```python
from build123d import *

# Parameters (mm, degrees)
SKETCH1_W                                         = 107.95
SKETCH1_H                                         = 101.6
SKETCH1_R                                         = 19.05
SKETCH1_R_2                                       = 2.15265
SKETCH1_W_2                                       = 6.604
SKETCH1_H_2                                       = 6.35
BOSS_EXTRUDE1_DEPTH                               = 6.604
F_10_32_TAPPED_HOLE1_D                            = 4.0386
F_10_32_TAPPED_HOLE1_DEPTH                        = 12.0396
F_10_32_TAPPED_HOLE1_TIP                          = 1.213317848
FILLET1_R                                         = 6.35
CSK_FOR_8_FLAT_HEAD_SOCKET_CAP_SCREW2_D           = 4.3053
CSK_FOR_8_FLAT_HEAD_SOCKET_CAP_SCREW2_CSINK_D     = 9.1186
CSK_FOR_8_FLAT_HEAD_SOCKET_CAP_SCREW2_CSINK_ANGLE = 82


with BuildPart() as part:
    # Sketch1 → Boss-Extrude1 (new body)
    with BuildSketch(Plane(origin=(0, 0, 0), x_dir=(0, 0, -1), z_dir=(1, 0, 0))):
        Rectangle(SKETCH1_W, SKETCH1_H)
        Circle(SKETCH1_R, mode=Mode.SUBTRACT)
        with Locations((-44.45, 31.75)):
            Circle(SKETCH1_R_2, mode=Mode.SUBTRACT)
        with Locations((-44.45, -31.75)):
            Circle(SKETCH1_R_2, mode=Mode.SUBTRACT)
        with Locations((44.45, 31.75)):
            Circle(SKETCH1_R_2, mode=Mode.SUBTRACT)
        with Locations((44.45, -31.75)):
            Circle(SKETCH1_R_2, mode=Mode.SUBTRACT)
        with Locations((-44.45, 41.275)):
            Rectangle(SKETCH1_W_2, SKETCH1_H_2, mode=Mode.SUBTRACT)
        with Locations((-44.45, 22.225)):
            Rectangle(SKETCH1_W_2, SKETCH1_H_2, mode=Mode.SUBTRACT)
        with Locations((-44.45, -22.225)):
            Rectangle(SKETCH1_W_2, SKETCH1_H_2, mode=Mode.SUBTRACT)
        with Locations((-44.45, -41.275)):
            Rectangle(SKETCH1_W_2, SKETCH1_H_2, mode=Mode.SUBTRACT)
        with Locations((44.45, 41.275)):
            Rectangle(SKETCH1_W_2, SKETCH1_H_2, mode=Mode.SUBTRACT)
        with Locations((44.45, 22.225)):
            Rectangle(SKETCH1_W_2, SKETCH1_H_2, mode=Mode.SUBTRACT)
        with Locations((44.45, -41.275)):
            Rectangle(SKETCH1_W_2, SKETCH1_H_2, mode=Mode.SUBTRACT)
        with Locations((44.45, -22.225)):
            Rectangle(SKETCH1_W_2, SKETCH1_H_2, mode=Mode.SUBTRACT)
    extrude(amount=BOSS_EXTRUDE1_DEPTH)

    # #10-32 Tapped Hole1
    with Locations(Plane(origin=(6.604, 0, 0), x_dir=(0, 0, -1), z_dir=(1, 0, 0))):
        with Locations((-23.622, 23.622), (23.622, 23.622), (-23.622, -23.622), (23.622, -23.622)):
            Hole(F_10_32_TAPPED_HOLE1_D / 2, depth=F_10_32_TAPPED_HOLE1_DEPTH)
            with Locations((0, 0, -(F_10_32_TAPPED_HOLE1_DEPTH + F_10_32_TAPPED_HOLE1_TIP / 2))):  # 118° drill point
                Cone(0, F_10_32_TAPPED_HOLE1_D / 2, F_10_32_TAPPED_HOLE1_TIP, mode=Mode.SUBTRACT)

    # Fillet1
    fillet1_edges = [part.edges().sort_by_distance(p)[0] for p in [
        (3.302, -50.8, -53.975),
        (3.302, -50.8, 53.975),
        (3.302, 50.8, 53.975),
        (3.302, 50.8, -53.975),
    ]]
    fillet(fillet1_edges, radius=FILLET1_R)

    # CSK for #8 Flat Head Socket Cap Screw2 (through all)
    with Locations(Plane.ZY):
        with Locations((-44.45, 31.75), (-23.622, 23.622), (23.622, 23.622), (44.45, 31.75), (23.622, -23.622), (-23.622, -23.622), (-44.45, -31.75), (44.45, -31.75)):
            CounterSinkHole(CSK_FOR_8_FLAT_HEAD_SOCKET_CAP_SCREW2_D / 2, CSK_FOR_8_FLAT_HEAD_SOCKET_CAP_SCREW2_CSINK_D / 2, counter_sink_angle=CSK_FOR_8_FLAT_HEAD_SOCKET_CAP_SCREW2_CSINK_ANGLE)


solid = part.part
```
Input: part model. Units: mm. Frame: model coordinates. A direction names the side the tool comes from. Round coordinates to 2 decimals unless told otherwise and drop trailing zeros. Loops run counter-clockwise (first coordinate to the right, second up) from the corner with the lowest first, then second, coordinate; pieces in that order, holes last. Notation, with made-up numbers: (-1.75, 17) -> (25.25, 17) arc R30 ccw to (25.25, 54) -> close; hole circle Ø7 at (78.25, -4.5). An arc over 180 degrees is marked (long way). Write each question's results on one line, items separated by ' | '.
1. Section A-A (z = -44.45). State how many separate pieces and enclosed holes the cut face has, and give its area (3 significant figures).
Geometry results:
separate pieces: 7 | enclosed holes: 0 | area: 433 mm2
2. Section B-B (y = -31.75). Return loops of the section in (x, z) (3 decimals).
Geometry results:
outline: (0, -53.975) -> (6.604, -53.975) -> (6.604, -46.603) -> (2.769, -46.603) -> (0, -49.009) -> close; (0, -39.891) -> (2.769, -42.297) -> (6.604, -42.297) -> (6.604, 42.297) -> (2.769, 42.297) -> (0, 39.891) -> close; (0, 49.009) -> (2.769, 46.603) -> (6.604, 46.603) -> (6.604, 53.975) -> (0, 53.975) -> close
3. Set-up query: faces 4 (the face through (0, 1, 25)), 5 (the face through (3, -41, 41.148)). Return all of +Z, -Z, +X, -X, +Y, -Y with unobstructed straight access to the full face (end or side cutting, diameter ignored); none if empty.
Geometry results:
face 4: +Z, -Z, -X, +Y, -Y | face 5: +X, -X
4. Section D-D (y = 14.5). Return loops of the section in (x, z) (3 decimals).
Geometry results:
outline: (0, -53.975) -> (6.604, -53.975) -> (6.604, -12.355) -> (0, -12.355) -> close; (0, 12.355) -> (6.604, 12.355) -> (6.604, 53.975) -> (0, 53.975) -> close
5. Mould query, pull axis Z, two halves, no side actions, for faces 1 (the face through (6.604, 1, 25)), 2 (the face through (3.348, 48.89, 52.164)), 3 (the face through (3, 44.45, 44)). Classes: +Z half, -Z half, draft (parallel to the pull), parting line (faces both ways), or undercut.
Geometry results:
face 1: draft | face 2: +Z half | face 3: undercut
6. Section C-C (z = 11). Return loops of the section in (x, y).
Geometry results:
outline: (0, -50.8) -> (6.6, -50.8) -> (6.6, -15.55) -> (0, -15.55) -> close; (0, 15.55) -> (6.6, 15.55) -> (6.6, 50.8) -> (0, 50.8) -> close
7. Ray query, line 1 (Z direction, x = 2.25, y = 40) (3 decimals); line 2 (Z direction, x = 5.7, y = 31.75) (3 decimals); line 3 (Y direction, x = 0.5, z = 0). Return the intervals inside material, ascending. Write a range as from..to.
Geometry results:
line 1: -53.975..-47.752, -41.148..41.148, 47.752..53.975 | line 2: -53.975..-46.603, -42.297..42.297, 46.603..53.975 | line 3: -50.8..-19.05, 19.05..50.8
